The model under review builds one solid part; all positions refer to its coordinate system, in mm. Give positions to 0.01 mm unless a question says otherwise; leave off trailing zeros. Order: outer loops, then holes, each group sorted by start corner. A loop starts at its lowest first (then second) coordinate and runs counter-clockwise, first axis right, second up. Notation, with made-up numbers: (4.25, -39.5) -> (51.25, -39.5) arc R12 cw to (51.25, -31.5) -> close; hole circle Ø1 at (-3, -26). An arc over 180 degrees is marked (long way). Use one line per item in the form item = value.
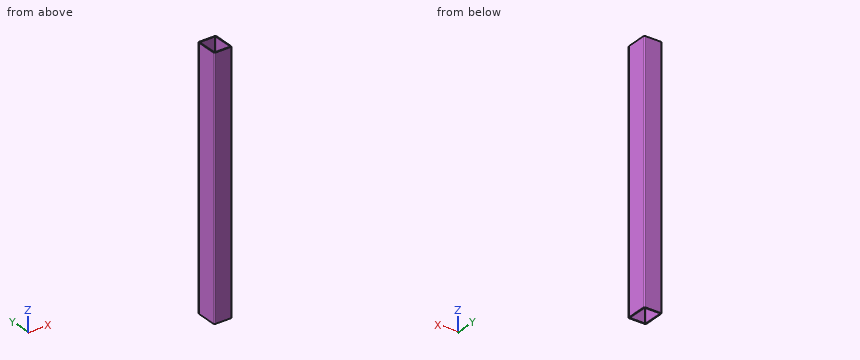
Autodesk Inventor part; units mm, degrees
ref_plane "Start plane" through (0, 0, 40) normal (0, 0, 1) x (1, 0, 0)
ref_plane "End plane" through (0, 0, 611) normal (0, 0, 1) x (1, 0, 0)
ref_plane "Work Plane4" through (20, 22, 40) normal (0, 0, -1) x (-1, 0, 0)
ref_plane "Start plane" through (0, 0, 40) normal (0, 0, 1) x (1, 0, 0)
ref_plane "End plane" through (0, 0, 611) normal (0, 0, 1) x (1, 0, 0)
sketch "Sketch" plane through (0, 0, 0) normal (0, 0, 1) x (1, 0, 0)
  line L0 (-20, -22) -> (-20, 22)
  line L1 (-17, 25) -> (17, 25)
  line L2 (20, 22) -> (20, -22)
  line L3 (17, -25) -> (-17, -25)
  arc A0 (-20, -22) -> (-17, -25) centre (-17, -22) ccw
  arc A1 (-17, 25) -> (-20, 22) centre (-17, 22) ccw
  arc A2 (20, 22) -> (17, 25) centre (17, 22) ccw
  arc A3 (17, -25) -> (20, -22) centre (17, -22) ccw
  arc A4 (-17, 23) -> (-18, 22) centre (-17, 22) ccw
  line L4 (-17, 23) -> (17, 23)
  arc A5 (18, 22) -> (17, 23) centre (17, 22) ccw
  line L5 (18, 22) -> (18, -22)
  arc A6 (17, -23) -> (18, -22) centre (17, -22) ccw
  line L6 (17, -23) -> (-17, -23)
  arc A7 (-18, -22) -> (-17, -23) centre (-17, -22) ccw
  line L7 (-18, -22) -> (-18, 22)
  line L8 (0, 35.8698) -> (0, -35.8698) construction
  line L9 (-28.8698, 0) -> (28.8698, 0) construction
  dimension "d7" = 3
  dimension "d10" = 50
  dimension "d11" = 40
  dimension "d12" = 2
  dimension "d15" = 25
  dimension "d16" = 20
extrude "Body" add sketch "Sketch" along normal up to surface (571 mm away) from surface at 40
sketch "Sketch3" plane through (0, 0, 0) normal (0, 0, 1) x (1, 0, 0)
  line L0 (0, 0) -> (10, 0)
ref_plane "Work Plane3" through (0, 0, 0) normal (0, -1, 0) x (1, 0, 0)
sketch "Sketch4" plane through (0, 0, 0) normal (0, -1, 0) x (1, 0, 0)
  line L0 (-2, 40) -> (12, 40)
  line L1 (-2, 611) -> (12, 611)
  dimension "d18" = 571
ref_plane "Work Plane4" through (20, 22, 40) normal (0, 0, -1) x (-1, 0, 0)
split "Split1" plane through (20, 22, 40) removes the side toward (0, 0, -1)
ref_plane "Work Plane5" through (20, -22, 611) normal (0, 0, 1) x (1, 0, 0)
split "Split2" plane through (20, -22, 611) removes the side toward (0, 0, 1)
equation "\"d7\" = G_IR"
equation "\"d10\" = G_H"
equation "\"d11\" = G_W"
equation "\"d12\" = G_T"
equation "\"d15\" = 0.5 * d10"
equation "\"d16\" = 0.5 * d11"
equation "\"d3\" = G_L"
equation "\"G_W\" = 40"
equation "\"G_H\" = 50"
equation "\"G_T\" = 2"
equation "\"G_IR\" = 3"
equation "\"G_L\" = d18"
equation "\"G_OFFSET_START\" = -40"
equation "\"G_OFFSET_END\" = -40"
equation "\"d13\" = -G_OFFSET_START"
equation "\"d14\" = G_OFFSET_END + B_L"
equation "\"B_L\" = 651"
properties part number "UNI EN 10305-5 - 50 x 40 x 2  - 571" material "Steel, Mild"
1. Add section B-B on x = 2.5. Give the boundary of the cut face in (y, z), then the cut area to 3 significant figures.
Values:
outline = (-25, 40) -> (-23, 40) -> (-23, 611) -> (-25, 611) -> close; (23, 40) -> (25, 40) -> (25, 611) -> (23, 611) -> close
area = 2,280 mm^2
2. For L1, parallel to Y at x = 17, z = 463; L2, parallel to X at y = 19.5, z = 228, list the stretches that pass through material, from the lowest coordinate up.
Values:
L1 = -25 to -23, 23 to 25
L2 = -20 to -18, 18 to 20
3. Add section C-C on z = 178. Give the boundary of the cut face in (x, y), then the cut area to 3 significant figures.
Values:
outline = (-20, -22) arc R3 ccw to (-17, -25) -> (17, -25) arc R3 ccw to (20, -22) -> (20, 22) arc R3 ccw to (17, 25) -> (-17, 25) arc R3 ccw to (-20, 22) -> close; hole (-18, -22) arc R1 ccw to (-17, -23) -> (17, -23) arc R1 ccw to (18, -22) -> (18, 22) arc R1 ccw to (17, 23) -> (-17, 23) arc R1 ccw to (-18, 22) -> close
area = 337 mm^2
4. Add section A-A on y = 16. Give the boundary of the cut face in (x, z), then the cut area to 3 significant figures.
Values:
outline = (-20, 40) -> (-18, 40) -> (-18, 611) -> (-20, 611) -> close; (18, 40) -> (20, 40) -> (20, 611) -> (18, 611) -> close
area = 2,280 mm^2
